Design review of the part built by this model. Coordinates are the model's own, in mm. Face numbers are marked on the shaded views. A direction names the side the tool comes from. Coordinates: 2 decimals unless noted, no trailing zeros. Loops run counter-clockwise (first coordinate to the right, second up) from the corner with the lowest first, then second, coordinate; pieces in that order, holes last. Notation, with made-up numbers: (-33.5, 14.5) -> (11.5, 14.5) arc R13 ccw to (11.5, 25.5) -> close; hole circle Ø9 at (-5, 78.5). An arc over 180 degrees is marked (long way). Answer as a JSON object with one key per item and string values.
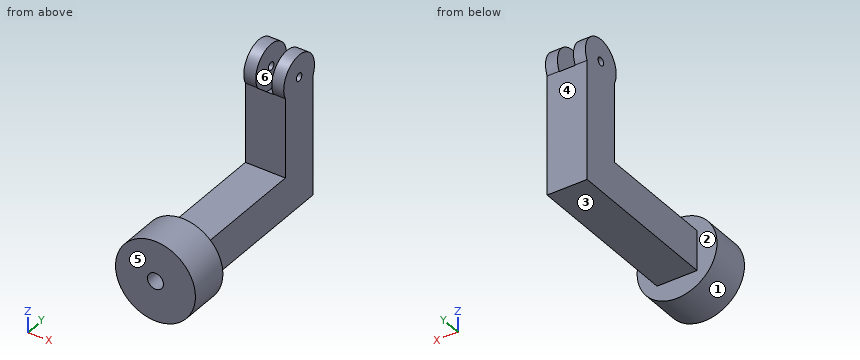
```python
from build123d import *

# Parameters (mm, degrees)
SKETCH1_R               = 25
BOSS_EXTRUDE1_DEPTH     = 25
SKETCH2_W               = 25
SKETCH2_H               = 25
BOSS_EXTRUDE2_DEPTH     = 100
SKETCH7_R               = 5
CUT_EXTRUDE2_DEPTH      = 10
SKETCH8_W               = 25
SKETCH8_H               = 25
BOSS_EXTRUDE3_DEPTH     = 50
SKETCH10_R              = 14
BOSS_EXTRUDE4_DEPTH     = 12.5
SKETCH13_R              = 14.15
CUT_EXTRUDE4_DEPTH      = 5
CUT_EXTRUDE5_DEPTH      = 154.080044421
CUT_EXTRUDE5_DEPTH_BACK = 154.080044421
SKETCH14_R              = 2.5


with BuildPart() as part:
    # Sketch1 → Boss-Extrude1 (new body)
    with BuildSketch(Plane(origin=(0, 0, 0), x_dir=(1, 0, 0), z_dir=(0, 1, 0))):
        with Locations(Location((0, 0, 0), (0, 0, 270))):
            Circle(SKETCH1_R)
    extrude(amount=BOSS_EXTRUDE1_DEPTH)

    # Sketch2 → Boss-Extrude2 (add)
    with BuildSketch(Plane(origin=(0, 25, 0), x_dir=(1, 0, 0), z_dir=(0, 1, 0))):
        Rectangle(SKETCH2_W, SKETCH2_H)
    extrude(amount=BOSS_EXTRUDE2_DEPTH)

    # Sketch7 → Cut-Extrude2 (cut)
    with BuildSketch(Plane.XZ):
        with Locations(Location((0, 0, 0), (0, 0, 270))):
            Circle(SKETCH7_R)
    extrude(amount=-CUT_EXTRUDE2_DEPTH, mode=Mode.SUBTRACT)

    # Sketch8 → Boss-Extrude3 (add)
    with BuildSketch(Plane.XY.offset(12.5)):
        with Locations((0, 112.5)):
            Rectangle(SKETCH8_W, SKETCH8_H)
    extrude(amount=BOSS_EXTRUDE3_DEPTH)

    # Sketch10 → Boss-Extrude4 (add, symmetric)
    with BuildSketch(Plane(origin=(0, 0, 0), x_dir=(0, 0, -1), z_dir=(1, 0, 0))):
        with Locations((-68.5, 112.5)):
            Circle(SKETCH10_R)
    extrude(amount=BOSS_EXTRUDE4_DEPTH, both=True)

    # Sketch13 → Cut-Extrude4 (cut, symmetric)
    with BuildSketch(Plane(origin=(0, 0, 0), x_dir=(0, 0, -1), z_dir=(1, 0, 0))):
        with Locations((-68.595239894, 112.5)):
            Circle(SKETCH13_R)
    extrude(amount=CUT_EXTRUDE4_DEPTH, both=True, mode=Mode.SUBTRACT)

    # Sketch14 → Cut-Extrude5 (cut, two sides: drawn at the far end of the back side and taken through both)
    with BuildSketch(Plane(origin=(0, 0, 0), x_dir=(0, 0, -1), z_dir=(1, 0, 0)).offset(-CUT_EXTRUDE5_DEPTH_BACK)):
        with Locations((-68.595239894, 112.5)):
            Circle(SKETCH14_R)
    extrude(amount=CUT_EXTRUDE5_DEPTH + CUT_EXTRUDE5_DEPTH_BACK, mode=Mode.SUBTRACT)


solid = part.part
```
1) Add section A-A, the plane y = 112.5. Give the boundary of the cut face in (x, z).
Completed:
{"outline": "(-12.5, -12.5) -> (12.5, -12.5) -> (12.5, 66.1) -> (5, 66.1) -> (5, 54.45) -> (-5, 54.45) -> (-5, 66.1) -> (-12.5, 66.1) -> close; (-12.5, 71.1) -> (-5, 71.1) -> (-5, 82.5) -> (-12.5, 82.5) -> close; (5, 71.1) -> (12.5, 71.1) -> (12.5, 82.5) -> (5, 82.5) -> close"}
2) The part is to be moulded in two halves that separate along Y. For the marked faces 4, 5 and 6, say which applies: pulls with the +Y half, pulls with the -Y half, needs draft (parallel to the pull), parting line crosses it, or undercut.
Completed:
{"face 4": "pulls with the +Y half", "face 5": "pulls with the -Y half", "face 6": "undercut"}
3) Wall thickness on probe 1 along X at (y, z) = (5.25, 0); probe 2 along X at (y, z) = (102.5, 63.5); probe 3 along Y at (x, z) = (-6, 51): over which ranges is each line inside the solid? List them lowest first.
Completed:
{"probe 1": "-25 to -5, 5 to 25", "probe 2": "-12.5 to -5, 5 to 12.5", "probe 3": "100 to 125"}
4) Add section D-D, the plane z = 68.5. Give the boundary of the cut face in (x, y).
Completed:
{"outline": "(-12.5, 98.5) -> (-5, 98.5) -> (-5, 110) -> (-12.5, 110) -> close; (-12.5, 115) -> (-5, 115) -> (-5, 126.5) -> (-12.5, 126.5) -> close; (5, 98.5) -> (12.5, 98.5) -> (12.5, 110) -> (5, 110) -> close; (5, 115) -> (12.5, 115) -> (12.5, 126.5) -> (5, 126.5) -> close"}
5) Clearance check with flat-ended pins moving along their axes: pin 1 Ø6 at (y, z) = (112.5, 68.6) entering from -X; pin 2 Ø7.5 at (x, z) = (0.5, 36.5) entering from -Y; pin 3 Ø12 at (x, y) = (17.5, 25) entering from -Z; pin 4 Ø8 at (x, z) = (18, 29.5) entering from -Y. State where each tip first meets the part, or that it passes through.
Completed:
{"pin 1": "x = -12.5", "pin 2": "y = 100", "pin 3": "z = -22.2", "pin 4": "through"}
6) Add section B-B, the plane z = 0. Give the boundary of the cut face in (x, y), and give its area (3 significant figures).
Completed:
{"outline": "(-25, 0) -> (-5, 0) -> (-5, 10) -> (5, 10) -> (5, 0) -> (25, 0) -> (25, 25) -> (12.5, 25) -> (12.5, 125) -> (-12.5, 125) -> (-12.5, 25) -> (-25, 25) -> close", "area": "3,650 mm²"}
7) For the marked faces 1, 2 and 3, list the 3-axis set-ups (+Z, -Z, +X, -X, +Y, -Y) from which the entire face can be reached by the end or side of a thin tool; tool diameter is ignored.
Completed:
{"face 1": "-Y", "face 2": "none", "face 3": "-Z, +X, -X, +Y"}
8) Add section C-C, the plane x = 0. Give the boundary of the cut face in (y, z), and give its area (3 significant figures).
Completed:
{"outline": "(0, -25) -> (25, -25) -> (25, -12.5) -> (125, -12.5) -> (125, 61.96) arc R14.15 cw to (100, 61.96) -> (100, 12.5) -> (25, 12.5) -> (25, 25) -> (0, 25) -> (0, 5) -> (10, 5) -> (10, -5) -> (0, -5) -> close", "area": "4,750 mm²"}
